The listing builds one solid part. Answer for the finished solid, in the listing's coordinates (mm). A direction names the side the tool comes from. Coordinates: 2 decimals unless noted, no trailing zeros. Loops run counter-clockwise (first coordinate to the right, second up) from the corner with the lowest first, then second, coordinate; pieces in that order, holes last. Notation, with made-up numbers: (36, 73.5) - (94, 73.5) arc R19 cw to (94, 95.5) - close; hole circle Ø2 at (68, 64). An arc over 180 degrees is marked (long way). Put each result on its own line as item: value.
```python
from build123d import *

# Parameters (mm, degrees)
SKETCH1_W           = 43.6
SKETCH1_H           = 34
BOSS_EXTRUDE1_DEPTH = 2
SKETCH2_W           = 43.6
SKETCH2_H           = 2
BOSS_EXTRUDE2_DEPTH = 35.8
SKETCH3_W           = 12.2
SKETCH3_H           = 29.71
CUT_EXTRUDE2_DEPTH  = 66.8
CUT_EXTRUDE3_DEPTH  = 66.8


with BuildPart() as part:
    # Sketch1 → Boss-Extrude1 (new body)
    with BuildSketch(Plane(origin=(0, 0, 0), x_dir=(1, 0, 0), z_dir=(0, 1, 0))):
        Rectangle(SKETCH1_W, SKETCH1_H)
    extrude(amount=BOSS_EXTRUDE1_DEPTH)

    # Sketch2 → Boss-Extrude2 (add)
    with BuildSketch(Plane(origin=(0, 2, 0), x_dir=(1, 0, 0), z_dir=(0, 1, 0))):
        with Locations((0, 16)):
            Rectangle(SKETCH2_W, SKETCH2_H)
        with Locations((0, -16)):
            Rectangle(SKETCH2_W, SKETCH2_H)
    extrude(amount=BOSS_EXTRUDE2_DEPTH)

    # Sketch3 → Cut-Extrude2 (cut)
    with BuildSketch(Plane.XY.offset(17)):
        with Locations((-6.1, 22.945)):
            Rectangle(SKETCH3_W, SKETCH3_H)
        with Locations((6.1, 22.945)):
            Rectangle(SKETCH3_W, SKETCH3_H)
    extrude(amount=-CUT_EXTRUDE2_DEPTH, mode=Mode.SUBTRACT)

    # Sketch4 → Cut-Extrude3 (cut)
    with BuildSketch(Plane(origin=(0, 2, 0), x_dir=(1, 0, 0), z_dir=(0, 1, 0))):
        with BuildLine():
            ThreePointArc((-3.75, 5), (-5.883883476, 5.883883476), (-5, 3.75))
            Line((-5, 3.75), (-5, 5))
            Line((-5, 5), (-3.75, 5))
        make_face()
        with BuildLine():
            Line((-5, 5), (-5, 3.75))
            ThreePointArc((-5, 3.75), (-4.116116524, 4.116116524), (-3.75, 5))
            Line((-3.75, 5), (-5, 5))
        make_face()
        with BuildLine():
            ThreePointArc((3.75, 5), (4.116116524, 4.116116524), (5, 3.75))
            Line((5, 3.75), (5, 5))
            Line((5, 5), (3.75, 5))
        make_face()
        with BuildLine():
            Line((5, 5), (5, 3.75))
            ThreePointArc((5, 3.75), (5.883883476, 4.116116524), (6.25, 5))
            ThreePointArc((6.25, 5), (5, 6.25), (3.75, 5))
            Line((3.75, 5), (5, 5))
        make_face()
        with BuildLine():
            Line((-5, -3.75), (-5, -5))
            Line((-5, -5), (-3.75, -5))
            ThreePointArc((-3.75, -5), (-4.116116524, -4.116116524), (-5, -3.75))
        make_face()
        with BuildLine():
            Line((-3.75, -5), (-5, -5))
            Line((-5, -5), (-5, -3.75))
            ThreePointArc((-5, -3.75), (-5.883883476, -5.883883476), (-3.75, -5))
        make_face()
        with BuildLine():
            ThreePointArc((5, -3.75), (4.116116524, -4.116116524), (3.75, -5))
            Line((3.75, -5), (5, -5))
            Line((5, -5), (5, -3.75))
        make_face()
        with BuildLine():
            Line((5, -5), (3.75, -5))
            ThreePointArc((3.75, -5), (5, -6.25), (6.25, -5))
            ThreePointArc((6.25, -5), (5.883883476, -4.116116524), (5, -3.75))
            Line((5, -3.75), (5, -5))
        make_face()
    extrude(amount=-CUT_EXTRUDE3_DEPTH, mode=Mode.SUBTRACT)


solid = part.part
```
1) The part is cut by section C-C (z = -12). Give the vertices of the cut face in (x, y).
Found:
outline: (-21.8, 0) - (21.8, 0) - (21.8, 2) - (-21.8, 2) - close
2) The part is cut by section D-D (x = -15.5). Give the vertices of the cut face in (y, z), and give its area (3 significant figures).
Found:
outline: (0, -17) - (37.8, -17) - (37.8, -15) - (2, -15) - (2, 15) - (37.8, 15) - (37.8, 17) - (0, 17) - close
area: 211 mm^2
3) The part is cut by section B-B (x = 10). Give the vertices of the cut face in (y, z), and give its area (3 significant figures).
Found:
outline: (0, -17) - (8.09, -17) - (8.09, -15) - (2, -15) - (2, 15) - (8.09, 15) - (8.09, 17) - (0, 17) - close
area: 92.4 mm^2
4) The part is cut by section A-A (y = 11.5). Give the vertices of the cut face in (x, z), and give its area (3 significant figures).
Found:
outline: (-21.8, -17) - (-12.2, -17) - (-12.2, -15) - (-21.8, -15) - close; (-21.8, 15) - (-12.2, 15) - (-12.2, 17) - (-21.8, 17) - close; (12.2, -17) - (21.8, -17) - (21.8, -15) - (12.2, -15) - close; (12.2, 15) - (21.8, 15) - (21.8, 17) - (12.2, 17) - close
area: 76.8 mm^2
5) Straight lines are drawn through the part: L1, parallel to Z at x = -5, y = 1.65; L2, parallel to X at y = 0.55, z = 5; L3, parallel to Z at x = 15, y = 29.5. For each, find the intervals that lie inside material, in ascending order. Write a range as [from, to].
Found:
L1: z = [-17, -6.25], [-3.75, 3.75], [6.25, 17]
L2: x = [-21.8, -6.25], [-3.75, 3.75], [6.25, 21.8]
L3: z = [-17, -15], [15, 17]
6) For faces 5 (the face through (0, 8.09, 16)), 6 (the face through (17, 37.8, -16)), 7 (the face through (0, 2, 0)), determine the directions among +Z, -Z, +X, -X, +Y, -Y from which every point of the face is accessible in a straight line to the end or side of a thin tool.
Found:
face 5: +Z, -Z, +Y
face 6: +Z, -Z, +X, -X, +Y
face 7: +X, -X, +Y
7) Each of these flat-tipped pins is pushed along its axis until it touches: pin 1 (2 mm diameter, centred on x = 3, z = 16, fed in from +Y); pin 2 (2 mm diameter, centred on x = -10.5, z = -12, fed in from +Y). Where does it stop, or does it pass through?
Found:
pin 1: stops at y = 8.09
pin 2: stops at y = 2
8) For a pull along Z with two mould halves and no side action, classify faces 1 (the face through (0, 6, 17)), 2 (the face through (-0.3, 7.7, -15)), 3 (the face through (-21.8, 16, 15.2)), 4 (the face through (-0.3, 7.7, 15)) as pulls with the +Z half, pulls with the -Z half, needs draft (parallel to the pull), parting line crosses it, or undercut.
Found:
face 1: pulls with the +Z half
face 2: undercut
face 3: needs draft
face 4: undercut
